```python
from build123d import *

# Parameters (mm, degrees)
BOSS_EXTRU_1_DEPTH      = 15.25
ESQUISSE2_W             = 250.5
ESQUISSE2_H             = 135
ENL_V_MAT_EXTRU_1_DEPTH = 10
ESQUISSE3_W             = 15.75
ESQUISSE3_H             = 29.857142857
ESQUISSE3_H_2           = 29.857142858
ENL_V_MAT_EXTRU_2_DEPTH = 15.25


with BuildPart() as part:
    # Esquisse1 → Boss.-Extru.1 (new body)
    with BuildSketch(Plane(origin=(0, 0, 0), x_dir=(1, 0, 0), z_dir=(0, 1, 0))):
        Polygon((-113.085152838, 185.313864629), (-163.085152838, 185.313864629), (-163.085152838, -20.186135371), (167.414847162, -20.186135371), (167.414847162, 185.313864629), (117.414847162, 185.313864629), (117.414847162, 60.313864629), (-113.085152838, 60.313864629), align=None)
    extrude(amount=BOSS_EXTRU_1_DEPTH)

    # Esquisse2 → Enlèv. mat.-Extru.1 (cut)
    with BuildSketch(Plane(origin=(0, 15.25, 0), x_dir=(1, 0, 0), z_dir=(0, 1, 0))):
        with Locations((2.164847162, 117.813864629)):
            Rectangle(ESQUISSE2_W, ESQUISSE2_H)
    extrude(amount=-ENL_V_MAT_EXTRU_1_DEPTH, mode=Mode.SUBTRACT)

    # Esquisse3 → Enlèv. mat.-Extru.2 (cut)
    with BuildSketch(Plane(origin=(0, 15.25, 0), x_dir=(1, 0, 0), z_dir=(0, 1, 0))):
        with Locations((-155.210152838, 170.385293201)):
            Rectangle(ESQUISSE3_W, ESQUISSE3_H)
        with Locations((-155.210152838, 111.837674152)):
            Rectangle(ESQUISSE3_W, ESQUISSE3_H)
        with Locations((-155.210152838, 53.290055105)):
            Rectangle(ESQUISSE3_W, ESQUISSE3_H_2)
        with Locations((-155.210152838, -5.257563943)):
            Rectangle(ESQUISSE3_W, ESQUISSE3_H)
    enl_v_mat_extru_2 = extrude(amount=-ENL_V_MAT_EXTRU_2_DEPTH, mode=Mode.SUBTRACT)

    # Symétrie1: Enlèv. mat.-Extru.2 across plane
    add(enl_v_mat_extru_2.mirror(Plane.ZY.offset(-2.164847162)), mode=Mode.SUBTRACT)


solid = part.part
```
Work out the finished part from the listing and answer in its coordinate system (mm). A direction names the side the tool comes from. Coordinates: 2 decimals unless noted, no trailing zeros. Write each loop counter-clockwise with the first axis right and the second up, starting at its lowest first coordinate (ties: lowest second). Pieces come first, ordered by that corner, then holes. Notation, with made-up numbers: (-15, -15.5) - (26, -15.5) arc R15 cw to (26, -10.5) - close; hole circle Ø5 at (21, 71). An arc over 180 degrees is marked (long way). Answer as a JSON object with one key per item and string values.
Q1. Find section A-A (z = -112.5). Write down the section's boundary in (x, y), plus the area to 3 significant figures.
Results list:
{"outline": "(-147.34, 0) - (-113.09, 0) - (-113.09, 5.25) - (-123.09, 5.25) - (-123.09, 15.25) - (-147.34, 15.25) - close; (117.41, 0) - (151.66, 0) - (151.66, 15.25) - (127.41, 15.25) - (127.41, 5.25) - (117.41, 5.25) - close", "area": "845 mm^2"}
Q2. For a pull along X with two mould halves and no side action, classify faces 4 (the flat face through (0, 10, -50.314)), 5 (the flat face through (-134, 8, -185.314)), 6 (the flat face through (-147.335, 8, -112)), 7 (the flat face through (-123.085, 10, -117)) as pulls with the +X half, pulls with the -X half, needs draft (parallel to the pull), parting line crosses it, or undercut.
Results list:
{"face 4": "undercut", "face 5": "needs draft", "face 6": "pulls with the -X half", "face 7": "undercut"}
Q3. Which of the six approach directions +Z, -Z, +X, -X, +Y, -Y give full straight-line access (tool end or side, diameter ignored) to faces 1 (the flat face through (151.665, 8, -170)), 2 (the flat face through (-147.335, 8, -170)), 3 (the flat face through (160, 8, -126.766))?
Results list:
{"face 1": "-Z, +X, +Y, -Y", "face 2": "-Z, -X, +Y, -Y", "face 3": "+X, +Y, -Y"}
Q4. Find section C-C (x = -90). Write down the section's boundary in (y, z).
Results list:
{"outline": "(0, -60.31) - (5.25, -60.31) - (5.25, -50.31) - (15.25, -50.31) - (15.25, 20.19) - (0, 20.19) - close"}
Q5. Find section D-D (z = 6.5). Write down the section's boundary in (x, y).
Results list:
{"outline": "(-147.34, 0) - (151.66, 0) - (151.66, 15.25) - (-147.34, 15.25) - close"}
Q6. Consider L1, parallel to X at y = 10.75, z = -99; L2, parallel to X at y = 11, z = -146.5; L3, parallel to X at y = 12.5, z = -3. Determine where each line is inside the solid, lowest interval first. Write a range as from..to.
Results list:
{"L1": "x = -147.34..-123.09, 127.41..151.66", "L2": "x = -163.09..-123.09, 127.41..167.41", "L3": "x = -147.34..151.66"}
Q7. Given pin 1 Ø7.5 at (x, y) = (162, 9) entering from -Z; pin 2 Ø7.5 at (x, y) = (161, 5.5) entering from +Z; pin 3 Ø7.5 at (y, z) = (5, -114.5) entering from -X, each flat-ended and moving along its own axis, determine where each tip first touches the part or whether it passes through.
Results list:
{"pin 1": "stops at z = -155.46", "pin 2": "stops at z = -9.67", "pin 3": "stops at x = -147.34"}
